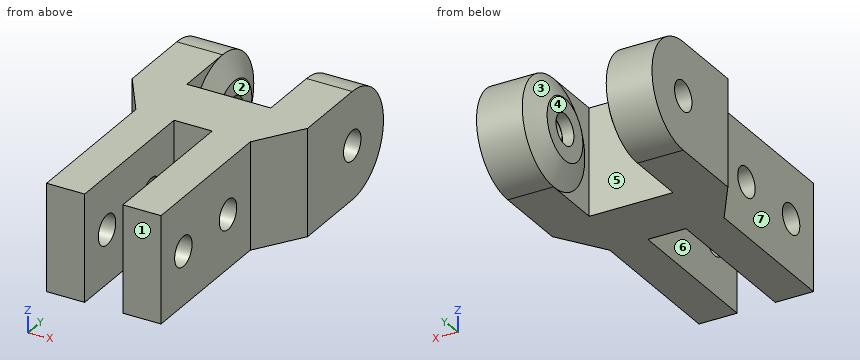
```python
from build123d import *

# Parameters (mm, degrees)
BOSS_EXTRUDE1_DEPTH = 3.5
SKETCH2_R           = 0.975
CUT_EXTRUDE1_DEPTH  = 7.5


with BuildPart() as part:
    # Sketch1 → Boss-Extrude1 (new body, symmetric)
    with BuildSketch(Plane.XY):
        Polygon((-1.25, -10), (-3.75, -10), (-3.75, 0), (-5.75, 3), (-5.75, 12), (-4.25, 12), (-2.75, 12), (-2.75, 4), (2.75, 4), (2.75, 12), (4.25, 12), (5.75, 12), (5.75, 3), (3.75, 0), (3.75, -10), (1.25, -10), (1.25, 0), (-1.25, 0), align=None)
    extrude(amount=BOSS_EXTRUDE1_DEPTH, both=True)

    # Sketch2 → Cut-Extrude1 (cut, symmetric)
    with BuildSketch(Plane(origin=(0, 0, 0), x_dir=(0, 0, -1), z_dir=(1, 0, 0))):
        with BuildLine():
            Line((-3.5, 12), (-3.5, 7.991246091))
            ThreePointArc((-3.5, 7.991246091), (0, 11.491246091), (3.5, 7.991246091))
            Line((3.5, 7.991246091), (3.5, 12))
            Line((3.5, 12), (-3.5, 12))
        make_face()
        with Locations((0, 7.991246091)):
            Circle(SKETCH2_R)
        with Locations((0, -2.5)):
            Circle(SKETCH2_R)
        with Locations((0, -7.5)):
            Circle(SKETCH2_R)
    extrude(amount=CUT_EXTRUDE1_DEPTH, both=True, mode=Mode.SUBTRACT)

    # Sketch3 → Revolve1 (revolve)
    with BuildSketch(Plane.XY):
        Polygon((-2.75, 8.991246091), (-2, 8.991246091), (-2, 9.991246091), (-2.75, 11.491246091), align=None)
    revolve1 = revolve(axis=Axis((-5.75, 7.991246091, 0), (1, 0, 0)))

    # Mirror1: Revolve1 across plane
    add(revolve1.mirror(Plane(origin=(0, 0, 0), x_dir=(0, 0, 1), z_dir=(1, 0, 0))))


solid = part.part
```
Geometry check sheet. Reference: the model listing, model coordinates, mm. Face numbers are marked on the shaded views. A direction names the side the tool comes from. Give positions to 0.01 mm unless a question says otherwise; leave off trailing zeros. Order: outer loops, then holes, each group sorted by start corner. A loop starts at its lowest first (then second) coordinate and runs counter-clockwise, first axis right, second up.
1. Gauge pin test, flat ends, axial feed: pin 1 Ø3 at (y, z) = (8.5, -0.5) entering from +X; pin 2 Ø2 at (y, z) = (-6, 1) entering from -X; pin 3 Ø1 at (x, z) = (1, 2) entering from +Y; pin 4 Ø2 at (y, z) = (-0.5, 2.5) entering from -X. Record the tip position at first contact, or that the pin passes through.
2. Section check A-A, the plane x = 2.25. Enter the section's corners in (y, z) (3 decimals), and give its area (3 significant figures).
3. Section check D-D, the plane y = -6.75. Enter the section's corners in (x, z), and give its area (3 significant figures).
4. Release check for a two-part mould opening along Y. For the marked faces 1, 2 and 3 record: pulls with the +Y half, pulls with the -Y half, needs draft (parallel to the pull), parting line crosses it, or undercut.
5. Access from +Z, -Z, +X, -X, +Y, -Y to the whole of each face (thin tool, end or side, straight path). Record for the marked faces 4, 5, 6 and 7.
6. Section check C-C, the plane z = 0. Give the number of separate pieces and of enclosed holes in the cut face, and give its area (3 significant figures).
7. Thickness scan on L1, parallel to Y at x = 3.1, z = 0 (3 decimals); L2, parallel to Y at x = -1.9, z = 0 (3 decimals); L3, parallel to Z at x = 2.5, y = -2.5 (3 decimals). Record the ranges inside material, lowest first.
8. Section check B-B, the plane y = -2.5. Enter the section's corners in (x, z) (3 decimals).
Values follow:
1. pin 1: stops at x = 5.75
1. pin 2: stops at x = -3.75
1. pin 3: stops at y = 4
1. pin 4: stops at x = -4.08
2. outline: (-10, -3.5) - (4, -3.5) - (4, 3.5) - (-10, 3.5) - close; circle Ø5 at (7.991, 0); hole circle Ø1.95 at (-7.5, 0); hole circle Ø1.95 at (-2.5, 0); hole circle Ø2 at (7.991, 0)
2. area: 109 mm2
3. outline: (-3.75, -3.5) - (-1.25, -3.5) - (-1.25, -0.62) - (-3.75, -0.62) - close; (-3.75, 0.62) - (-1.25, 0.62) - (-1.25, 3.5) - (-3.75, 3.5) - close; (1.25, -3.5) - (3.75, -3.5) - (3.75, -0.62) - (1.25, -0.62) - close; (1.25, 0.62) - (3.75, 0.62) - (3.75, 3.5) - (1.25, 3.5) - close
3. area: 28.8 mm2
4. face 1: pulls with the -Y half
4. face 2: needs draft
4. face 3: undercut
5. face 4: +Z, -Z, +Y
5. face 5: +Z, -Z
5. face 6: +Z, -Z, -Y
5. face 7: +Z, -Z, -X, -Y
6. separate pieces: 7
6. enclosed holes: 0
6. area: 109 mm2
7. L1: y = -10 to -8.475, -6.525 to -3.475, -1.525 to 7.016, 8.966 to 11.491
7. L2: y = -10 to -8.475, -6.525 to -3.475, -1.525 to 4
7. L3: z = -3.5 to -0.975, 0.975 to 3.5
8. outline: (-3.75, -3.5) - (-1.25, -3.5) - (-1.25, -0.975) - (-3.75, -0.975) - close; (-3.75, 0.975) - (-1.25, 0.975) - (-1.25, 3.5) - (-3.75, 3.5) - close; (1.25, -3.5) - (3.75, -3.5) - (3.75, -0.975) - (1.25, -0.975) - close; (1.25, 0.975) - (3.75, 0.975) - (3.75, 3.5) - (1.25, 3.5) - close
